The listing builds one solid part. Answer for the finished solid, in the listing's coordinates (mm). A direction names the side the tool comes from. Round coordinates to 2 decimals unless told otherwise and drop trailing zeros. Write each loop counter-clockwise with the first axis right and the second up, starting at its lowest first coordinate (ties: lowest second). Pieces come first, ordered by that corner, then holes. Notation, with made-up numbers: (22.25, 14) - (33.25, 14) arc R16 cw to (33.25, 23) - close; hole circle Ø4 at (-9.75, 41). An arc over 180 degrees is marked (long way). Return JSON: item names as keys, results as strings. Group by question number.
(1) This flat-tipped pin is pushed along its axis until it touches: pin 1 (1.6 mm diameter, centred on x = 37.338, z = 0, fed in from -Y). Where does it stop, or does it pass through?
(2) Determine the mould class of faces 4 (the cylindrical face through (38.68, -80, 0.18)), 5 (the flat face through (37.382, -32.194, -34.381)), 6 (the cylindrical face through (37.857, -76.293, -10.011)) for opening direction X: +X half, -X half, draft (parallel to the pull), parting line (faces both ways), or undercut.
(3) Section D-D, the plane y = -40.5 is taken. Write down the section's boundary in (x, z) (3 decimals).
(4) Section C-C, the plane z = 43 is taken. Write down the section's boundary in (x, y), then the cut area to 3 significant figures.
(5) Section A-A, the plane x = -25.4 is taken. Write down the section's boundary in (y, z) (3 decimals).
(6) Section B-B, the plane y = -52 is taken. Write down the section's boundary in (x, z), then the cut area to 3 significant figures.
(7) Find the intervals of material crossed by line 1 along Z through (x, y) = (25, 3); line 2 along X through (y, z) = (4.25, -38.1) (3 decimals); line 3 along X through (y, z) = (-79.9, 0), in increasing order. Write a range as [from, to].
(8) Which of the six approach directions +Z, -Z, +X, -X, +Y, -Y give full straight-line access (tool end or side, diameter ignored) to faces 1 (the flat face through (-34.163, -22, 1)), 2 (the cylindrical face through (-38.68, -80, 0.18)), 3 (the flat face through (-37.382, -32.194, -34.381))?
```python
from build123d import *

# Parameters (mm, degrees)
SKETCH2_W               = 81.026
SKETCH2_H               = 101.6
BOSS_EXTRUDE1_DEPTH     = 6.35
SKETCH3_R               = 14.605
BOSS_EXTRUDE2_DEPTH     = 6.35
SKETCH5_R               = 1.35255
CUT_EXTRUDE1_DEPTH      = 16.256
SKETCH6_R               = 1.35255
CUT_EXTRUDE2_DEPTH      = 9.652
MIRROR2_COPY_1_SKETCH_R = 1.35255
MIRROR2_COPY_1_DEPTH    = 9.652
SKETCH7_R               = 3.175
CUT_EXTRUDE3_DEPTH      = 6.35


with BuildPart() as part:
    # Sketch2 → Boss-Extrude1 (new body)
    with BuildSketch(Plane(origin=(0, 0, 0), x_dir=(1, 0, 0), z_dir=(0, 1, 0))):
        Rectangle(SKETCH2_W, SKETCH2_H)
    extrude(amount=BOSS_EXTRUDE1_DEPTH)

    # Sketch3 → Boss-Extrude2 (add)
    with BuildSketch(Plane(origin=(40.513, 0, 0), x_dir=(0, 0, -1), z_dir=(1, 0, 0))):
        with BuildLine():
            Line((-50.8, 6.35), (-50.8, 0))
            Line((-50.8, 0), (-18.415, -63.5))
            ThreePointArc((-18.415, -63.5), (0, -81.915), (18.415, -63.5))
            Line((18.415, -63.5), (50.8, 0))
            Line((50.8, 0), (50.8, 6.35))
            Line((50.8, 6.35), (-50.8, 6.35))
        make_face()
        with Locations((0, -63.5)):
            Circle(SKETCH3_R, mode=Mode.SUBTRACT)
    boss_extrude2 = extrude(amount=-BOSS_EXTRUDE2_DEPTH)

    # Sketch5 → Cut-Extrude1 (cut)
    with BuildSketch(Plane(origin=(0, -81.915, 0), x_dir=(-1, 0, 0), z_dir=(0, -1, 0))):
        with Locations(Location((-37.338, 0, 0), (0, 0, 90))):
            Circle(SKETCH5_R)
    cut_extrude1 = extrude(amount=-CUT_EXTRUDE1_DEPTH, mode=Mode.SUBTRACT)

    # Sketch6 → Cut-Extrude2 (cut)
    with BuildSketch(Plane(origin=(0, -45.669396988, -45.669396988), x_dir=(1, 0, 0), z_dir=(0, 0.7071067811865464, 0.7071067811865488))):
        with Locations(Location((37.339349705, -48.118027143, 0), (0, 0, 90))):
            Circle(SKETCH6_R)
    cut_extrude2 = extrude(amount=CUT_EXTRUDE2_DEPTH, mode=Mode.SUBTRACT)

    # Mirror1: Cut-Extrude2 across plane
    add(cut_extrude2.mirror(Plane.XY), mode=Mode.SUBTRACT)

    # Mirror2: Boss-Extrude2, Cut-Extrude1, Cut-Extrude2 across plane
    add(boss_extrude2.mirror(Plane(origin=(0, 0, 0), x_dir=(0, 0, 1), z_dir=(1, 0, 0))))
    add(cut_extrude1.mirror(Plane(origin=(0, 0, 0), x_dir=(0, 0, 1), z_dir=(1, 0, 0))), mode=Mode.SUBTRACT)
    add(cut_extrude2.mirror(Plane(origin=(0, 0, 0), x_dir=(0, 0, 1), z_dir=(1, 0, 0))), mode=Mode.SUBTRACT)

    # Mirror2 copy 1 sketch → Mirror2 copy 1 (cut)
    with BuildSketch(Plane(origin=(0, -45.669396988, 45.669396988), x_dir=(-1, 0, 0), z_dir=(0, 0.7071067811865464, -0.7071067811865488))):
        with Locations(Location((37.339349705, -48.118027143, 0), (0, 0, 90))):
            Circle(MIRROR2_COPY_1_SKETCH_R)
    extrude(amount=MIRROR2_COPY_1_DEPTH, mode=Mode.SUBTRACT)

    # Sketch7 → Cut-Extrude3 (cut)
    with BuildSketch(Plane.XZ):
        with Locations(Location((-25.4, 38.1, 0), (0, 0, 270))):
            Circle(SKETCH7_R)
        with Locations(Location((25.4, 38.1, 0), (0, 0, 270))):
            Circle(SKETCH7_R)
        with Locations(Location((25.4, -38.1, 0), (0, 0, 270))):
            Circle(SKETCH7_R)
        with Locations(Location((-25.4, -38.1, 0), (0, 0, 270))):
            Circle(SKETCH7_R)
    extrude(amount=-CUT_EXTRUDE3_DEPTH, mode=Mode.SUBTRACT)


solid = part.part
```
Working result:
{
 "1": {"pin 1": "stops at y = -48.92"},
 "2": {"face 4": "undercut", "face 5": "draft", "face 6": "undercut"},
 "3": {"outline": "(-40.513, -30.145) - (-34.163, -30.145) - (-34.163, 30.145) - (-40.513, 30.145) - close; (34.163, -30.145) - (40.513, -30.145) - (40.513, 30.145) - (34.163, 30.145) - close"},
 "4": {"outline": "(-40.51, -15.29) - (-34.16, -15.29) - (-34.16, 0) - (34.16, 0) - (34.16, -15.29) - (40.51, -15.29) - (40.51, 6.35) - (-40.51, 6.35) - close", "area": "709 mm^2"},
 "5": {"outline": "(0, -50.8) - (6.35, -50.8) - (6.35, -41.275) - (0, -41.275) - close; (0, -34.925) - (6.35, -34.925) - (6.35, 34.925) - (0, 34.925) - close; (0, 41.275) - (6.35, 41.275) - (6.35, 50.8) - (0, 50.8) - close"},
 "6": {"outline": "(-40.51, -24.28) - (-34.16, -24.28) - (-34.16, -9) - (-40.51, -9) - close; (-40.51, 9) - (-34.16, 9) - (-34.16, 24.28) - (-40.51, 24.28) - close; (34.16, -24.28) - (40.51, -24.28) - (40.51, -9) - (34.16, -9) - close; (34.16, 9) - (40.51, 9) - (40.51, 24.28) - (34.16, 24.28) - close", "area": "388 mm^2"},
 "7": {"line 1": "z = [-50.8, -41.25], [-34.95, 34.95], [41.25, 50.8]", "line 2": "x = [-40.513, -28.575], [-22.225, 22.225], [28.575, 40.513]", "line 3": "x = [-40.51, -38.69], [-35.99, -34.16], [34.16, 35.99], [38.69, 40.51]"},
 "8": {"face 1": "+Z, -Z, -Y", "face 2": "-Y", "face 3": "-Z, +X, -X, -Y"}
}
